Geometry: see drawing. Coordinates: mm, zero at the bounding-box minimum. A direction names the side the tool comes from. Round coordinates to 2 decimals unless told otherwise and drop trailing zeros. Write each loop counter-clockwise with the first axis right and the second up, starting at its lowest first coordinate (ties: lowest second). Pieces come first, ordered by that corner, then holes. Notation, with made-up numbers: (83, 0.25) - (129, 0.25) arc R15 cw to (129, 26.25) - close; hole circle Ø5 at (45, 78). An arc over 180 degrees is marked (long way). Use a Markdown table: item, result. Add a question column.
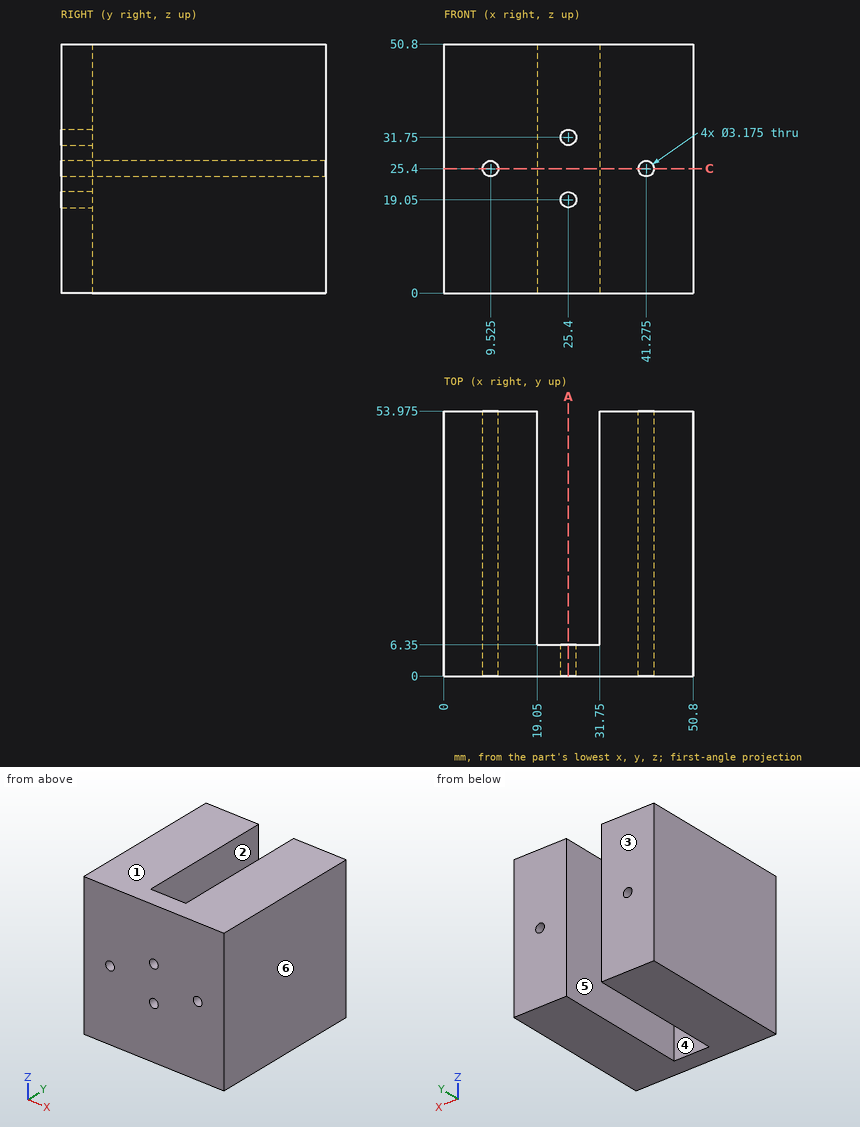
1) Section A-A, the plane x = 25.4. Return the cut outline in (y, z), then the cut area to 3 significant figures.
2) Section C-C, the plane z = 25.4. State how many separate pieces and enclosed holes the cut face has, then the cut area to 3 significant figures.
3) Pin query (flat end, axial travel): P1, Ø4, axis at x = 28, z = 37.5, coming from the +Y side. Return the tip coordinate at first contact, or that it passes through.
4) Material intervals for L1, parallel to X at y = 22.5, z = 25.4; L2, parallel to X at y = 36.5, z = 28.5; L3, parallel to X at y = 4.5, z = 19.05, sorted ascending. Write a range as from..to.
5) Draft query along X for the marked faces 3, 4, 5 and 6. Return one class per face: released by +X, released by -X, zero draft, split by the parting line, or undercut.
6) Set-up query: the marked faces 1 and 2. Return all of +Z, -Z, +X, -X, +Y, -Y with unobstructed straight access to the full face (end or side cutting, diameter ignored); none if empty.
Output values:
| question | item | result |
|---|---|---|
| 1 | outline | (0, 0) - (6.35, 0) - (6.35, 17.46) - (0, 17.46) - close; (0, 20.64) - (6.35, 20.64) - (6.35, 30.16) - (0, 30.16) - close; (0, 33.34) - (6.35, 33.34) - (6.35, 50.8) - (0, 50.8) - close |
| 1 | area | 282 mm^2 |
| 2 | separate pieces | 3 |
| 2 | enclosed holes | 0 |
| 2 | area | 1,790 mm^2 |
| 3 | P1 | stops at y = 6.35 |
| 4 | L1 | x = 0..7.94, 11.11..19.05, 31.75..39.69, 42.86..50.8 |
| 4 | L2 | x = 0..19.05, 31.75..50.8 |
| 4 | L3 | x = 0..23.81, 26.99..50.8 |
| 5 | face 3 | zero draft |
| 5 | face 4 | undercut |
| 5 | face 5 | undercut |
| 5 | face 6 | released by +X |
| 6 | face 1 | +Z, +X, -X, +Y, -Y |
| 6 | face 2 | +Z, -Z, +Y |
